Input: part model. Units: mm. Frame: model coordinates. A direction names the side the tool comes from. Give positions to 0.01 mm unless a question says otherwise; leave off trailing zeros. Loops run counter-clockwise (first coordinate to the right, second up) from the corner with the lowest first, then second, coordinate; pieces in that order, holes last. Notation, with made-up numbers: (29.5, 27) - (42.5, 27) arc R22 ccw to (42.5, 46) - close; hole circle Ø7 at (14.5, 9). An arc over 180 degrees is marked (long way). One line per item, written item: value.
Autodesk Fusion 360 part; units mm, degrees
sketch "Sketch1" plane through (0, 0, 0) normal (0, 1, 0) x (1, 0, 0)
  line L0 (72.5, -45) -> (-72.5, -45)
  line L1 (-72.5, -45) -> (-72.5, 45)
  line L2 (-72.5, 45) -> (72.5, 45)
  line L3 (72.5, 45) -> (72.5, -45)
  line L4 (72.5, -45) -> (-72.5, 45) construction
  line L5 (-72.5, -45) -> (72.5, 45) construction
  dimension "d1" = 145
  dimension "d2" = 90
extrude "Extrude1" add sketch "Sketch1" along normal blind 10
sketch "Sketch2" plane through (0, 10, 0) normal (0, 1, 0) x (-1, 0, 0)
  line L0 (-72.5, -45) -> (72.5, -45)
  line L1 (72.5, -45) -> (72.5, 45)
  line L2 (72.5, 45) -> (-72.5, 45)
  line L3 (-72.5, 45) -> (-72.5, -45)
  line L4 (72.5, -45) -> (55, -45)
  line L5 (55, -45) -> (55, 45)
  line L6 (55, 45) -> (72.5, 45)
  line L7 (72.5, 45) -> (72.5, -45)
  line L8 (-72.5, -45) -> (-55, -45)
  line L9 (-55, -45) -> (-55, 45)
  line L10 (-55, 45) -> (-72.5, 45)
  line L11 (-72.5, 45) -> (-72.5, -45)
  line L12 (-62.5, 30) -> (62.5, 30) construction
  line L13 (62.5, 30) -> (62.5, -30) construction
  line L14 (62.5, -30) -> (-62.5, -30) construction
  line L15 (-62.5, -30) -> (-62.5, 30) construction
  line L16 (-62.5, 30) -> (62.5, -30) construction
  line L17 (62.5, 30) -> (-62.5, -30) construction
  circle A0 centre (62.5, 30) radius 5
  circle A1 centre (-62.5, 30) radius 5
  circle A2 centre (62.5, -30) radius 5
  circle A3 centre (-62.5, -30) radius 5
  line L18 (-40, 40) -> (40, 40)
  line L19 (40, 40) -> (40, -40)
  line L20 (40, -40) -> (-40, -40)
  line L21 (-40, -40) -> (-40, 40)
  line L22 (-40, 40) -> (40, -40) construction
  line L23 (40, 40) -> (-40, -40) construction
  line L24 (-27.5, 27.5) -> (27.5, 27.5)
  line L25 (27.5, 27.5) -> (27.5, -27.5)
  line L26 (27.5, -27.5) -> (-27.5, -27.5)
  line L27 (-27.5, -27.5) -> (-27.5, 27.5)
  line L28 (-27.5, 27.5) -> (27.5, -27.5) construction
  line L29 (27.5, 27.5) -> (-27.5, -27.5) construction
  line L30 (-40, 6) -> (40, 6) construction
  line L31 (40, 6) -> (40, -6) construction
  line L32 (40, -6) -> (-40, -6) construction
  line L33 (-40, -6) -> (-40, 6) construction
  line L34 (-40, 6) -> (40, -6) construction
  line L35 (40, 6) -> (-40, -6) construction
  line L36 (-40, -6) -> (-55, -6)
  line L37 (-55, -6) -> (-55, 6)
  line L38 (-55, 6) -> (-40, 6)
  line L39 (-40, 6) -> (-40, -6)
  line L40 (40, -6) -> (55, -6)
  line L41 (55, -6) -> (55, 6)
  line L42 (55, 6) -> (40, 6)
  line L43 (40, 6) -> (40, -6)
  dimension "d5" = 17.5
  dimension "d6" = 90
  dimension "d7" = 17.5
  dimension "d8" = 90
  dimension "d9" = 125
  dimension "d10" = 60
  dimension "d11" = 10
  dimension "d14" = -125
  dimension "d15" = -60
  dimension "d16" = 80
  dimension "d17" = 80
  dimension "d18" = 55
  dimension "d19" = 55
  dimension "d20" = 80
  dimension "d21" = 12
  dimension "d22" = 12
  dimension "d23" = 12
extrude "Extrude2" add sketch "Sketch2" along normal blind 30 contours L0 L2 L3 L8 L9 L10 L11 L37 | L0 L1 L2 L4 L5 L6 L7 L41 | L18 L19 L20 L21 L39 L43
extrude "Extrude3" cut sketch "Sketch2" against normal blind 10 contours A0 | A1 | A2 | A3
extrude "Extrude4" add sketch "Sketch2" along normal blind 10 contours L24 L25 L26 L27
extrude "Extrude5" add sketch "Sketch2" along normal blind 25 contours L9 L21 L36 L37 L38 L39 | L5 L19 L40 L41 L42 L43
sketch "Sketch3" plane through (0, 0, 0) normal (0, -1, 0) x (1, 0, 0)
  circle A0 centre (62.5, -30) radius 5
  circle A1 centre (-62.5, -30) radius 5
  circle A2 centre (62.5, 30) radius 5
  circle A3 centre (-62.5, 30) radius 5
  line L0 (-72.5, -45) -> (72.5, -45)
  line L1 (72.5, -45) -> (72.5, 45)
  line L2 (72.5, 45) -> (-72.5, 45)
  line L3 (-72.5, 45) -> (-72.5, -45)
  line L4 (30, 45) -> (-30, 45)
  line L5 (-30, 45) -> (-30, -45)
  line L6 (-30, -45) -> (30, -45)
  line L7 (30, -45) -> (30, 45)
  line L8 (30, 45) -> (-30, -45) construction
  line L9 (-30, 45) -> (30, -45) construction
  dimension "d32" = 60
  dimension "d33" = 90
extrude "Extrude6" add sketch "Sketch3" along normal blind 20 contours L0 L2 L4 L5 L6 L7
sketch "Sketch4" plane through (0, 20, 0) normal (0, 1, 0) x (-1, 0, 0)
  line L0 (-27.5, -27.5) -> (27.5, -27.5)
  line L1 (27.5, -27.5) -> (27.5, 27.5)
  line L2 (27.5, 27.5) -> (-27.5, 27.5)
  line L3 (-27.5, 27.5) -> (-27.5, -27.5)
  line L4 (-15, 15) -> (15, 15) construction
  line L5 (15, 15) -> (15, -15) construction
  line L6 (15, -15) -> (-15, -15) construction
  line L7 (-15, -15) -> (-15, 15) construction
  line L8 (-15, 15) -> (15, -15) construction
  line L9 (15, 15) -> (-15, -15) construction
  line L10 (10, -10) -> (20, -10)
  line L11 (20, -10) -> (20, -20)
  line L12 (20, -20) -> (10, -20)
  line L13 (10, -20) -> (10, -10)
  line L14 (10, -10) -> (20, -20) construction
  line L15 (20, -10) -> (10, -20) construction
  line L16 (-10, -20) -> (-20, -20)
  line L17 (-20, -20) -> (-20, -10)
  line L18 (-20, -10) -> (-10, -20) construction
  line L19 (-10, -10) -> (-10, -20)
  line L20 (-10, -10) -> (-20, -20) construction
  line L21 (-20, -10) -> (-10, -10)
  line L22 (20, 10) -> (10, 10)
  line L23 (10, 10) -> (10, 20)
  line L24 (10, 20) -> (20, 10) construction
  line L25 (20, 20) -> (20, 10)
  line L26 (20, 20) -> (10, 10) construction
  line L27 (10, 20) -> (20, 20)
  line L28 (-10, 10) -> (-20, 10)
  line L29 (-20, 10) -> (-20, 20)
  line L30 (-20, 20) -> (-10, 10) construction
  line L31 (-10, 20) -> (-10, 10)
  line L32 (-10, 20) -> (-20, 10) construction
  line L33 (-20, 20) -> (-10, 20)
  point P0 (15, -15)
  point P1 (-15, -15)
  point P2 (-15, -15)
  point P3 (15, 15)
  point P4 (15, 15)
  point P5 (-15, 15)
  point P6 (-15, 15)
  dimension "d36" = 30
  dimension "d37" = 30
  dimension "d38" = 10
  dimension "d39" = 10
  dimension "d42" = -30
  dimension "d43" = 30
extrude "Extrude7" cut sketch "Sketch4" against normal blind 40 contours L10 L11 L12 L13 | L16 L17 L19 L21 | L22 L23 L25 L27 | L28 L29 L31 L33
Item 1: Section B-B, the plane y = -6. Output: boundary loops of the cut face in (x, z).
Verdict:
outline: (-30, -45) - (30, -45) - (30, 45) - (-30, 45) - close; hole (-20, -20) - (-10, -20) - (-10, -10) - (-20, -10) - close; hole (-20, 10) - (-10, 10) - (-10, 20) - (-20, 20) - close; hole (10, -20) - (20, -20) - (20, -10) - (10, -10) - close; hole (10, 10) - (20, 10) - (20, 20) - (10, 20) - close
Item 2: Pin query (flat end, axial travel): P1, Ø8, axis at y = -7, z = -15, coming from the -X side; P2, Ø12, axis at x = -31, y = -11, coming from the -Z side; P3, Ø4, axis at y = -2.5, z = 34, coming from the +X side; P4, Ø6, axis at x = 62.5, z = -30, coming from the +Y side. Return the tip coordinate at first contact, or that it passes through.
Verdict:
P1: stops at x = -30
P2: stops at z = -45
P3: stops at x = 30
P4: passes through
Item 3: Material intervals for L1, parallel to Z at x = 62, y = 28; L2, parallel to X at y = 27.5, z = -10; L3, parallel to X at y = 14, z = -9, sorted ascending.
Verdict:
L1: z = -45 to -34.97, -25.03 to 25.03, 34.97 to 45
L2: x = -72.5 to -55, -40 to -27.5, 27.5 to 40, 55 to 72.5
L3: x = -72.5 to -55, -40 to 40, 55 to 72.5
Item 4: Section A-A, the plane z = 16. Output: boundary loops of the cut face in (x, y), and give its area (3 significant figures).
Verdict:
outline: (-72.5, 0) - (-30, 0) - (-30, -20) - (-20, -20) - (-20, 20) - (-27.5, 20) - (-27.5, 40) - (-40, 40) - (-40, 10) - (-55, 10) - (-55, 40) - (-72.5, 40) - close; (-10, -20) - (10, -20) - (10, 20) - (-10, 20) - close; (20, -20) - (30, -20) - (30, 0) - (72.5, 0) - (72.5, 40) - (55, 40) - (55, 10) - (40, 10) - (40, 40) - (27.5, 40) - (27.5, 20) - (20, 20) - close
area: 4,200 mm^2
Item 5: Access query for faces 1 (the face through (55, 25, 9)), 2 (the face through (-1, 25, -40)), 3 (the face through (30, -10, -1)), 4 (the face through (-15, 0, -10)). Directions: +Z, -Z, +X, -X, +Y, -Y. A direction counts if a zero-diameter tool reaches every point of the face in a straight line with its end or side. Return the directions, or none.
Verdict:
face 1: +Y
face 2: -Z, +Y
face 3: +Z, -Z, +X, -Y
face 4: +Y, -Y
Item 6: Draft query along X for faces 5 (the face through (72.5, 20, -1)), 6 (the face through (-55, 25, 9)), 7 (the face through (36, 40, 1)). Return one class per face: pulls with the +X half, pulls with the -X half, needs draft (parallel to the pull), parting line crosses it, or undercut.
Verdict:
face 5: pulls with the +X half
face 6: undercut
face 7: needs draft
Item 7: Section C-C, the plane x = -62.5. Output: boundary loops of the cut face in (y, z), and give its area (3 significant figures).
Verdict:
outline: (0, -45) - (40, -45) - (40, -35) - (0, -35) - close; (0, -25) - (40, -25) - (40, 25) - (0, 25) - close; (0, 35) - (40, 35) - (40, 45) - (0, 45) - close
area: 2,800 mm^2
Item 8: Section D-D, the plane y = 6. Count the separate pieces of the cut face and the enclosed holes in it, and give its area (3 significant figures).
Verdict:
separate pieces: 1
enclosed holes: 8
area: 12,300 mm^2
